The drawing under review shows one solid part. Ordinate dimensions are in mm from its lowest x, y, z. A direction names the side the tool comes from. Give positions to 0.01 mm unless a question says otherwise; leave off trailing zeros. Write each loop counter-clockwise with the first axis right and the second up, starting at its lowest first coordinate (ties: lowest second). Pieces come first, ordered by that corner, then holes. Notation, with made-up numbers: (22, 18.25) - (62, 18.25) arc R23 cw to (62, 52.25) - close; hole circle Ø7 at (-21.5, 19). An arc over 180 degrees is marked (long way). Write each question's results on one line, items separated by ' | '. Start each with the question number.
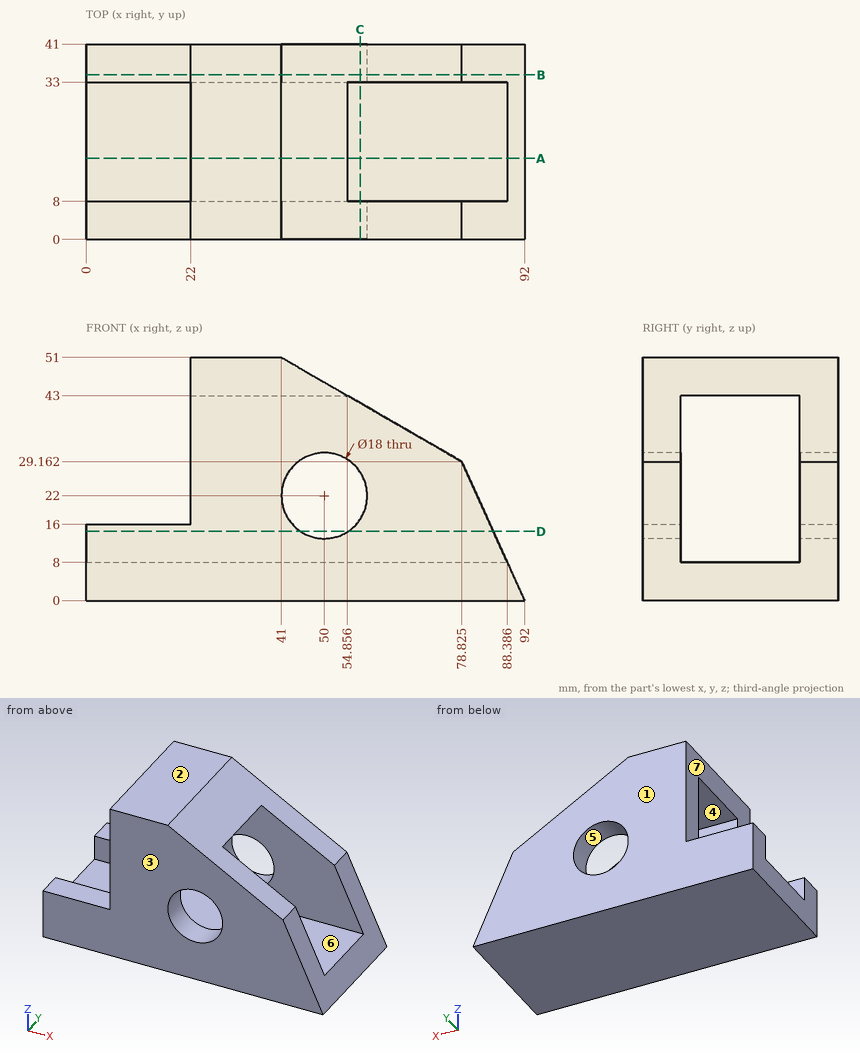
Q1. Machinability: for the marked faces 5, 6 and 7, which of the approach directions +Z, -Z, +X, -X, +Y, -Y give a long, thin tool a straight path to every point of the face, cutting with its end or side? Answer none if there is none.
Q2. The part is to be moulded in two halves that separate along Y. For the marked faces 1, 2, 3 and 4, say which applies: +Y half, -Y half, draft (parallel to the pull), parting line (faces both ways), or undercut.
Q3. Add section A-A on y = 17. State the section outline as (x, z) points (1 decimal).
Q4. Add section C-C on x = 57.5. State the section outline as (y, z) points (1 decimal).
Q5. Add section D-D on z = 14.5. State the section outline as (x, y) points (1 decimal), plus the area to 3 significant figures.
Q6. For line 1 along Z through (x, y) = (23.5, 31.5); line 2 along Y through (x, z) = (59, 15); line 3 along Z through (x, y) = (56, 11), list the stretches that pass through material, from the lowest coordinate up. Write a range as [from, to].
Q7. Insertion check: P1, Ø14.5, axis at x = 50, z = 22, coming from the +Y side; P2, Ø3, axis at x = 82, y = 7, coming from the +Z side (1 decimal); P3, Ø6.5, axis at x = 12, y = 5.5, coming from the +Z side; P4, Ø10, axis at x = 20, z = 19.5, coming from the +Y side. Each pin has a flat end and moves straight along its axis. Give the tip position at first contact, or say it passes through.
Q8. Add section B-B on y = 34.5. State the section outline as (x, z) points (1 decimal).
Result:
1) face 5: +Y, -Y | face 6: +X, -X | face 7: +Z, -X, +Y, -Y
2) face 1: +Y half | face 2: draft | face 3: -Y half | face 4: undercut
3) outline: (0, 0) - (92, 0) - (88.4, 8) - (0, 8) - close; (22, 43) - (54.9, 43) - (41, 51) - (22, 51) - close
4) outline: (0, 0) - (41, 0) - (41, 17) - (33, 17) - (33, 8) - (8, 8) - (8, 17) - (0, 17) - close; (0, 27) - (8, 27) - (8, 41.5) - (0, 41.5) - close; (33, 27) - (41, 27) - (41, 41.5) - (33, 41.5) - close
5) outline: (0, 0) - (45, 0) - (45, 8) - (0, 8) - close; (0, 33) - (45, 33) - (45, 41) - (0, 41) - close; (55, 0) - (85.4, 0) - (85.4, 8) - (55, 8) - close; (55, 33) - (85.4, 33) - (85.4, 41) - (55, 41) - close | area: 1,210 mm²
6) line 1: z = [0, 8], [43, 51] | line 2: y = [0, 8], [33, 41] | line 3: z = [0, 8]
7) P1: passes through | P2: stops at z = 25.5 | P3: stops at z = 16 | P4: stops at y = 41
8) outline: (0, 0) - (92, 0) - (78.8, 29.2) - (41, 51) - (22, 51) - (22, 16) - (0, 16) - close; hole circle Ø18 at (50, 22)
